from build123d import *

# Parameters (mm, degrees)
BOSS_EXTRUDE1_DEPTH  = 15
BOSS_EXTRUDE2_DEPTH  = 16
CUT_EXTRUDE1_DEPTH   = 1
SKETCH6_R            = 6.626408405
BOSS_EXTRUDE7_DEPTH  = 16
CUT_EXTRUDE3_DEPTH   = 10
SKETCH8_R            = 1.860980047
CUT_EXTRUDE6_DEPTH   = 1
BOSS_EXTRUDE10_DEPTH = 1
SKETCH10_R           = 1
CUT_EXTRUDE7_DEPTH   = 7
SKETCH11_R           = 1.75
CUT_EXTRUDE8_DEPTH   = 20
BOSS_EXTRUDE13_DEPTH = 1
SKETCH13_R           = 6
SKETCH13_R_2         = 7.350371073
SKETCH13_R_3         = 5.24539952
SKETCH13_R_4         = 2.694037488
BOSS_EXTRUDE14_DEPTH = 1
BOSS_EXTRUDE19_DEPTH = 0.2


with BuildPart() as part:
    # Sketch3 → Boss-Extrude1 (new body)
    with BuildSketch(Plane.XY):
        with BuildLine():
            Line((-50, 100), (50, 100))
            ThreePointArc((50, 100), (57.071067812, 97.071067812), (60, 90))
            Line((60, 90), (60, -90))
            ThreePointArc((60, -90), (57.071067812, -97.071067812), (50, -100))
            Line((50, -100), (-50, -100))
            ThreePointArc((-50, -100), (-57.071067812, -97.071067812), (-60, -90))
            Line((-60, -90), (-60, 90))
            ThreePointArc((-60, 90), (-57.071067812, 97.071067812), (-50, 100))
        make_face()
    extrude(amount=BOSS_EXTRUDE1_DEPTH)

    # Sketch4 → Boss-Extrude2 (add)
    with BuildSketch(Plane.XY):
        with BuildLine():
            Line((-45.696681728, 86.479793583), (45.696681728, 86.479793583))
            ThreePointArc((45.696681728, 86.479793583), (52.400974756, 83.702784485), (55.177983854, 76.998491457))
            Line((55.177983854, 76.998491457), (55.177983854, -76.998491457))
            ThreePointArc((55.177983854, -76.998491457), (52.400974756, -83.702784485), (45.696681728, -86.479793583))
            Line((45.696681728, -86.479793583), (-45.696681728, -86.479793583))
            ThreePointArc((-45.696681728, -86.479793583), (-52.400974756, -83.702784485), (-55.177983854, -76.998491457))
            Line((-55.177983854, -76.998491457), (-55.177983854, 76.998491457))
            ThreePointArc((-55.177983854, 76.998491457), (-52.400974756, 83.702784485), (-45.696681728, 86.479793583))
        make_face()
    extrude(amount=BOSS_EXTRUDE2_DEPTH)

    # Sketch5 → Cut-Extrude1 (cut)
    with BuildSketch(Plane.XY.offset(16)):
        with BuildLine():
            Line((-11.964009061, 76.758679218), (11.964009061, 76.758679218))
            ThreePointArc((11.964009061, 76.758679218), (18.133018595, 79.040091667), (21.333225963, 84.786411725))
            ThreePointArc((21.333225963, 84.786411725), (22.008282474, 85.998549041), (23.309582539, 86.479793583))
            Line((23.309582539, 86.479793583), (-7.969065225, 86.479793583))
            Line((-7.969065225, 86.479793583), (-23.309582539, 86.479793583))
            ThreePointArc((-23.309582539, 86.479793583), (-22.008282474, 85.998549041), (-21.333225963, 84.786411725))
            ThreePointArc((-21.333225963, 84.786411725), (-18.133018595, 79.040091667), (-11.964009061, 76.758679218))
        make_face()
    extrude(amount=-CUT_EXTRUDE1_DEPTH, mode=Mode.SUBTRACT)

    # Sketch6 → Boss-Extrude7 (add)
    with BuildSketch(Plane.XY):
        with Locations((-0.588195402, -93.239793583)):
            Circle(SKETCH6_R)
    extrude(amount=BOSS_EXTRUDE7_DEPTH)

    # Sketch7 → Cut-Extrude3 (cut)
    with BuildSketch(Plane.XZ.offset(100)):
        with BuildLine():
            Line((3.684816301, 6.392233542), (-2.315183699, 6.392233542))
            ThreePointArc((-2.315183699, 6.392233542), (-3.422950157, 7.5), (-2.315183699, 8.607766458))
            Line((-2.315183699, 8.607766458), (3.684816301, 8.607766458))
            ThreePointArc((3.684816301, 8.607766458), (4.792582759, 7.5), (3.684816301, 6.392233542))
        make_face()
    extrude(amount=-CUT_EXTRUDE3_DEPTH, mode=Mode.SUBTRACT)

    # Sketch8 → Cut-Extrude6 (cut)
    with BuildSketch(Plane.XY.offset(15)):
        with Locations((-10, 84.758679218)):
            Circle(SKETCH8_R)
        with BuildLine():
            Line((0, 85.758679218), (4, 85.758679218))
            ThreePointArc((4, 85.758679218), (5, 84.758679218), (4, 83.758679218))
            Line((4, 83.758679218), (0, 83.758679218))
            ThreePointArc((0, 83.758679218), (-1, 84.758679218), (0, 85.758679218))
        make_face()
    extrude(amount=-CUT_EXTRUDE6_DEPTH, mode=Mode.SUBTRACT)

    # Sketch9 → Boss-Extrude10 (add)
    with BuildSketch(Plane(origin=(60, 0, 0), x_dir=(0, 0, -1), z_dir=(1, 0, 0))):
        with BuildLine():
            Line((-5.280651792, 58.138580799), (-5.280651792, 43.138580799))
            ThreePointArc((-5.280651792, 43.138580799), (-7.5, 40.919232591), (-9.719348208, 43.138580799))
            Line((-9.719348208, 43.138580799), (-9.719348208, 58.138580799))
            ThreePointArc((-9.719348208, 58.138580799), (-7.5, 60.357929008), (-5.280651792, 58.138580799))
        make_face()
    extrude(amount=BOSS_EXTRUDE10_DEPTH)

    # Sketch10 → Cut-Extrude7 (cut)
    with BuildSketch(Plane.XZ.offset(100)):
        with Locations((-38.926720921, 7.5)):
            Circle(SKETCH10_R)
    extrude(amount=-CUT_EXTRUDE7_DEPTH, mode=Mode.SUBTRACT)

    # Sketch11 → Cut-Extrude8 (cut)
    with BuildSketch(Plane(origin=(0, 100, 0), x_dir=(1, 0, 0), z_dir=(0, 1, 0))):
        with Locations((-40.22365253, -7.5)):
            Circle(SKETCH11_R)
    extrude(amount=-CUT_EXTRUDE8_DEPTH, mode=Mode.SUBTRACT)

    # Sketch12 → Boss-Extrude13 (add)
    with BuildSketch(Plane(origin=(0, 0, 0), x_dir=(-1, 0, 0), z_dir=(0, 0, -1))):
        with BuildLine():
            Line((-18.925763354, 91.964241382), (-52.203053416, 91.964241382))
            ThreePointArc((-52.203053416, 91.964241382), (-55.738587322, 90.499775288), (-57.203053416, 86.964241382))
            Line((-57.203053416, 86.964241382), (-57.203053416, 52.022440164))
            ThreePointArc((-57.203053416, 52.022440164), (-55.738587322, 48.486906258), (-52.203053416, 47.022440164))
            Line((-52.203053416, 47.022440164), (-18.925763354, 47.022440164))
            ThreePointArc((-18.925763354, 47.022440164), (-15.390229448, 48.486906258), (-13.925763354, 52.022440164))
            Line((-13.925763354, 52.022440164), (-13.925763354, 86.964241382))
            ThreePointArc((-13.925763354, 86.964241382), (-15.390229448, 90.499775288), (-18.925763354, 91.964241382))
        make_face()
    extrude(amount=BOSS_EXTRUDE13_DEPTH)

    # Sketch13 → Boss-Extrude14 (add)
    with BuildSketch(Plane(origin=(0, 0, -1), x_dir=(-1, 0, 0), z_dir=(0, 0, -1))):
        with Locations((-48.871309333, 80.649061989)):
            Circle(SKETCH13_R)
        with Locations((-48.871309333, 55.649061989)):
            Circle(SKETCH13_R_2)
        with Locations((-28.684304458, 66.649061989)):
            Circle(SKETCH13_R_3)
        with Locations((-28.684304458, 80.649061989)):
            Circle(SKETCH13_R_4)
    extrude(amount=BOSS_EXTRUDE14_DEPTH)

    # Sketch14 → Boss-Extrude19 (add)
    with BuildSketch(Plane(origin=(0, 0, 0), x_dir=(-1, 0, 0), z_dir=(0, 0, -1))):
        with BuildLine():
            add(Edge.make_bspline(
                [(-3.674445913, 33.570119731), (-6.586996245, 36.726182993), (-9.97051323, 37.977315522), (-13.231414187, 37.431600611)],
                knots=[0.231070837, 0.231070837, 0.231070837, 0.231070837, 0.765352683, 0.765352683, 0.765352683, 0.765352683], degree=3))
            ThreePointArc((-13.231414187, 37.431600611), (-15.343951329, 36.616365238), (-17.406574019, 35.68201545))
            ThreePointArc((-17.406574019, 35.68201545), (-39.698794696, -0.448046182), (-16.596818278, -36.065782519))
            ThreePointArc((-16.596818278, -36.065782519), (-12.966582836, -36.280567352), (-10.151005098, -33.978988787))
            ThreePointArc((-10.151005098, -33.978988787), (0, -29.774304804), (10.151005098, -33.978988787))
            ThreePointArc((10.151005098, -33.978988787), (12.966582836, -36.280567352), (16.596818278, -36.065782519))
            ThreePointArc((16.596818278, -36.065782519), (18.986564068, -34.866967613), (21.29020582, -33.510031062))
            ThreePointArc((21.29020582, -33.510031062), (30.111316996, -25.874768297), (36.332224295, -16.005140531))
            ThreePointArc((36.332224295, -16.005140531), (20.757436471, 1.37873001), (33.896238409, 20.669786341))
            ThreePointArc((33.896238409, 20.669786341), (26.727072351, 29.357429199), (17.406574019, 35.68201545))
            ThreePointArc((17.406574019, 35.68201545), (15.343951329, 36.616365238), (13.231414187, 37.431600611))
            add(Edge.make_bspline(
                [(3.674445913, 33.570119731), (6.586996245, 36.726182993), (9.97051323, 37.977315522), (13.231414187, 37.431600611)],
                knots=[0.231070837, 0.231070837, 0.231070837, 0.231070837, 0.765352683, 0.765352683, 0.765352683, 0.765352683], degree=3))
            ThreePointArc((3.674445913, 33.570119731), (0, 31.961055772), (-3.674445913, 33.570119731))
        make_face()
        with BuildLine():
            ThreePointArc((13.231414187, 59.583781152), (11.301026929, 45.532102859), (0, 36.961055772))
            ThreePointArc((0, 36.961055772), (1.930387259, 51.012734065), (13.231414187, 59.583781152))
        make_face()
    extrude(amount=BOSS_EXTRUDE19_DEPTH)


solid = part.part
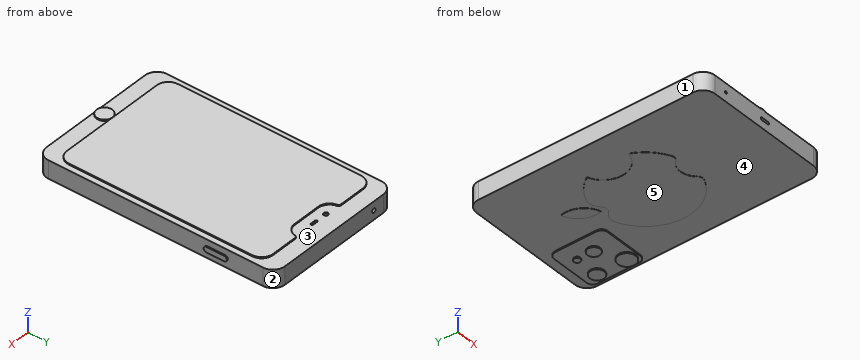
The listing builds one solid part. Answer for the finished solid, in the listing's coordinates (mm). Face numbers are marked on the shaded views. A direction names the side the tool comes from. Give positions to 0.01 mm unless a question says otherwise; leave off trailing zeros. Write each loop counter-clockwise with the first axis right and the second up, starting at its lowest first coordinate (ties: lowest second). Pieces come first, ordered by that corner, then holes. Notation, with made-up numbers: (-25, 19) -> (32, 19) arc R17 ccw to (32, 50) -> close; hole circle Ø8 at (-3.5, -29). An arc over 180 degrees is marked (long way). One line per question, with ' | ' between items. Start each with the question number.
1. Find the intervals of material crossed by probe 1 along X at (y, z) = (87, 7.5); probe 2 along X at (y, z) = (-79, 14.5); probe 3 along Z at (x, y) = (-40.5, 76), in increasing order.
2. For the marked faces 1, 2, 3, 4 and 5, determine the directions among +Z, -Z, +X, -X, +Y, -Y from which every point of the face is accessible in a straight line to the end or side of a thin tool.
3. Section B-B (y = -9) is taken. Determine the outline of the cut face in (x, z), plus the area to 3 significant figures.
4. Section A-A (y = -67.5) is taken. Determine the outline of the cut face in (x, z), plus the area to 3 significant figures.
5. Given pin 1 Ø12 at (x, y) = (-14.5, -19.5) entering from -Z; pin 2 Ø4 at (x, y) = (-9, 85) entering from +Z; pin 3 Ø0.5 at (x, y) = (60.5, 52.5) entering from -Z; pin 4 Ø4 at (x, z) = (-41, 7) entering from +Y, each flat-ended and moving along its own axis, determine where each tip first touches the part or whether it passes through.
Response values:
1) probe 1: -60 to -41.97, -38.47 to 60 | probe 2: -60 to 60 | probe 3: 0 to 16
2) face 1: +Z, -Z, -X, +Y, -Y | face 2: +Z, -Z, +X, +Y | face 3: +Z | face 4: -Z | face 5: -Z, +X, -X, -Y
3) outline: (-60, 0) -> (-24.71, 0) -> (-24.71, -0.2) -> (38.67, -0.2) -> (38.67, 0) -> (60, 0) -> (60, 15) -> (55.18, 15) -> (55.18, 16) -> (-55.18, 16) -> (-55.18, 15) -> (-60, 15) -> close | area: 1,920 mm2
4) outline: (-60, 0) -> (60, 0) -> (60, 15) -> (55.18, 15) -> (55.18, 16) -> (-55.18, 16) -> (-55.18, 15) -> (-60, 15) -> close | area: 1,910 mm2
5) pin 1: z = -0.2 | pin 2: z = 15 | pin 3: z = 5.28 | pin 4: y = 100
